The model under review builds one solid part; all positions refer to its coordinate system, in mm. A direction names the side the tool comes from. Round coordinates to 2 decimals unless told otherwise and drop trailing zeros. Order: outer loops, then holes, each group sorted by start corner. A loop starts at its lowest first (then second) coordinate and runs counter-clockwise, first axis right, second up. Notation, with made-up numbers: M 43.5,-32.5 L 50.5,-32.5 A12 ccw 50.5,-15.5 Z; hole C 63.5,87 d11. An arc over 180 degrees is marked long. Use a Markdown table: item, result. Add a question column.
1. The part is to be moulded in two halves that separate along Y. For faces 1 (the cylindrical face through (-2.57, 13.4, 19.79)), 2 (the flat face through (0, 20, 17)), 3 (the cylindrical face through (-7.43, 17.04, 8.44)), 4 (the cylindrical face through (7.91, 8.82, 2.46)), say which applies: +Y half, -Y half, draft (parallel to the pull), parting line (faces both ways), or undercut.
2. To check wall thickness, follow probe 1 along X at (y, z) = (7.5, 11); probe 2 along Y at (x, z) = (-10, 9.5); probe 3 along Z at (x, y) = (10.5, -12). State the ranges of each line that lie inside material, in increasing order.
3. Consider section C-C on z = 30. State the section outline as (x, y) points, then the cut area to 3 significant figures.
4. For faces 5 (the cylindrical face through (-2.57, -3.24, 5.6)), 6 (the cylindrical face through (7.986, 17.042, 31.586)), list the 3-axis set-ups (+Z, -Z, +X, -X, +Y, -Y) from which the entire face can be reached by the end or side of a thin tool; tool diameter is ignored.
5. Consider section A-A on y = 16. State the section outline as (x, z) points, then the cut area to 3 significant figures.
6. Consider section B-B on z = 23. State the section outline as (x, y) points, then the cut area to 3 significant figures.
7. Consider section D-D on x = 0.5. State the section outline as (y, z) points.
8. Insertion check: P1, Ø1.3, axis at x = 7.78, y = 7.78, coming from the -Z side; P2, Ø8, axis at x = -6.5, z = 18.5, coming from the -Y side; P3, Ø4, axis at x = -13, z = 22.5, coming from the -Y side; P4, Ø4, axis at x = 7, z = 15, coming from the -Y side. Each pin has a flat end and moves straight along its axis. Give the tip position at first contact, or say it passes through.
from build123d import *

# Parameters (mm, degrees)
SKETCH3_W                = 35
SKETCH3_H                = 40
BOSS_EXTRUDE1_DEPTH      = 5
SKETCH5_W                = 35
SKETCH5_H                = 30
BOSS_EXTRUDE2_DEPTH      = 6
BOSS_EXTRUDE3_DEPTH      = 4
BOSS_EXTRUDE4_DEPTH      = 2
BOSS_EXTRUDE4_DEPTH_BACK = 2
SKETCH9_R                = 1.05
CUT_EXTRUDE1_DEPTH       = 5
SKETCH10_R               = 1.6
CUT_EXTRUDE2_DEPTH       = 56.957573214
FILLET1_R                = 3
FILLET2_R                = 2


with BuildPart() as part:
    # Sketch3 → Boss-Extrude1 (new body)
    with BuildSketch(Plane.XY):
        Rectangle(SKETCH3_W, SKETCH3_H)
    extrude(amount=BOSS_EXTRUDE1_DEPTH)

    # Sketch5 → Boss-Extrude2 (add)
    with BuildSketch(Plane(origin=(0, 20, 0), x_dir=(1, 0, 0), z_dir=(0, 1, 0))):
        with Locations((0, -20)):
            Rectangle(SKETCH5_W, SKETCH5_H)
    extrude(amount=-BOSS_EXTRUDE2_DEPTH)

    # Sketch7 → Boss-Extrude3 (add)
    with BuildSketch(Plane(origin=(17.5, 0, 0), x_dir=(0, 0, -1), z_dir=(1, 0, 0))):
        Polygon((-35, 14), (-5, -20), (-5, 14), align=None)
    boss_extrude3 = extrude(amount=-BOSS_EXTRUDE3_DEPTH)

    # Mirror1: Boss-Extrude3 across plane
    add(boss_extrude3.mirror(Plane(origin=(0, 0, 0), x_dir=(0, 0, 1), z_dir=(1, 0, 0))))

    # Sketch8 → Boss-Extrude4 (add, two sides: drawn at the far end of the back side and taken through both)
    with BuildSketch(Plane(origin=(0, 0, 0), x_dir=(0, 0, -1), z_dir=(1, 0, 0)).offset(-BOSS_EXTRUDE4_DEPTH_BACK)):
        Polygon((-35, 14), (-5, -20), (-5, 14), align=None)
    extrude(amount=BOSS_EXTRUDE4_DEPTH + BOSS_EXTRUDE4_DEPTH_BACK)

    # Sketch9 → Cut-Extrude1 (cut)
    with BuildSketch(Plane(origin=(0, 0, 0), x_dir=(-1, 0, 0), z_dir=(0, 0, -1))):
        with Locations((-7.778174593, 7.778174593)):
            Circle(SKETCH9_R)
        with Locations((7.778174593, 7.778174593)):
            Circle(SKETCH9_R)
        with Locations((7.778174593, -7.778174593)):
            Circle(SKETCH9_R)
        with Locations((-7.778174593, -7.778174593)):
            Circle(SKETCH9_R)
    extrude(amount=-CUT_EXTRUDE1_DEPTH, mode=Mode.SUBTRACT)

    # Sketch10 → Cut-Extrude2 (cut, through all)
    with BuildSketch(Plane(origin=(0, 20, 0), x_dir=(1, 0, 0), z_dir=(0, 1, 0))):
        with Locations(Location((-7.778174593, -10, 0), (0, 0, 180))):
            Circle(SKETCH10_R)
        with Locations(Location((-7.778174593, -30, 0), (0, 0, 180))):
            Circle(SKETCH10_R)
        with Locations(Location((7.778174593, -30, 0), (0, 0, 180))):
            Circle(SKETCH10_R)
        with Locations(Location((7.778174593, -10, 0), (0, 0, 180))):
            Circle(SKETCH10_R)
    extrude(amount=-CUT_EXTRUDE2_DEPTH, mode=Mode.SUBTRACT)

    # Fillet1
    fillet1_edges = [part.edges().sort_by_distance(p)[0] for p in [
        (0, -20, 0),
        (-17.5, 0, 0),
        (17.5, 0, 0),
    ]]
    fillet(fillet1_edges, radius=FILLET1_R)

    # Fillet2
    # the kernel refuses this fillet: 2 mm, written as the material it adds along each edge
    with BuildSketch(Plane(origin=(13.5, 14, 0), x_dir=(0, -1, 0), z_dir=(0, 0, 1))) as fillet2_piece_1_section:
        with BuildLine():
            CenterArc((FILLET2_R, -FILLET2_R), FILLET2_R, 90, 90)
            Line((0, -FILLET2_R), (0, 0))
            Line((0, 0), (FILLET2_R, 0))
        make_face()
    fillet2_piece_1 = extrude(amount=35, mode=Mode.PRIVATE)
    fillet2_piece_1 = split(fillet2_piece_1, bisect_by=Plane(origin=(13.047209771, -2.378125245, 20.548713019), z_dir=(0, 0.6616216370868465, -0.7498378553650924)), keep=Keep.TOP, mode=Mode.PRIVATE)
    add(fillet2_piece_1)
    with BuildSketch(Plane(origin=(13.5, -20, 5), x_dir=(-1, 0, 0), z_dir=(0, 1, 0))) as fillet2_piece_2_section:
        with BuildLine():
            CenterArc((FILLET2_R, FILLET2_R), FILLET2_R, 180, 90)
            Line((0, FILLET2_R), (0, 0))
            Line((0, 0), (FILLET2_R, 0))
        make_face()
    fillet2_piece_2 = extrude(amount=39, mode=Mode.PRIVATE)
    fillet2_piece_2 = split(fillet2_piece_2, bisect_by=Plane(origin=(13.043521125, -10.077324079, 13.755302283), z_dir=(0, 0.6616216370868465, -0.7498378553650924)), keep=Keep.TOP, mode=Mode.PRIVATE)
    add(fillet2_piece_2)
    with BuildSketch(Plane(origin=(-13.5, 14, 0), x_dir=(0, -1, 0), z_dir=(0, 0, 1))) as fillet2_piece_3_section:
        with BuildLine():
            CenterArc((FILLET2_R, FILLET2_R), FILLET2_R, 180, 90)
            Line((0, FILLET2_R), (0, 0))
            Line((0, 0), (FILLET2_R, 0))
        make_face()
    fillet2_piece_3 = extrude(amount=35, mode=Mode.PRIVATE)
    fillet2_piece_3 = split(fillet2_piece_3, bisect_by=Plane(origin=(-13.047209771, -2.378125245, 20.548713019), z_dir=(0, 0.6616216370868465, -0.7498378553650924)), keep=Keep.TOP, mode=Mode.PRIVATE)
    add(fillet2_piece_3)
    with BuildSketch(Plane(origin=(-13.5, -20, 5), x_dir=(1, 0, 0), z_dir=(0, 1, 0))) as fillet2_piece_4_section:
        with BuildLine():
            CenterArc((FILLET2_R, -FILLET2_R), FILLET2_R, 90, 90)
            Line((0, -FILLET2_R), (0, 0))
            Line((0, 0), (FILLET2_R, 0))
        make_face()
    fillet2_piece_4 = extrude(amount=39, mode=Mode.PRIVATE)
    fillet2_piece_4 = split(fillet2_piece_4, bisect_by=Plane(origin=(-13.043521125, -10.077324079, 13.755302283), z_dir=(0, 0.6616216370868465, -0.7498378553650924)), keep=Keep.TOP, mode=Mode.PRIVATE)
    add(fillet2_piece_4)
    with BuildSketch(Plane(origin=(-2, 14, 0), x_dir=(-1, 0, 0), z_dir=(0, 0, 1))) as fillet2_piece_5_section:
        with BuildLine():
            CenterArc((FILLET2_R, FILLET2_R), FILLET2_R, 180, 90)
            Line((0, FILLET2_R), (0, 0))
            Line((0, 0), (FILLET2_R, 0))
        make_face()
    fillet2_piece_5 = extrude(amount=35, mode=Mode.PRIVATE)
    fillet2_piece_5 = split(fillet2_piece_5, bisect_by=Plane(origin=(-2.452790229, -2.378125245, 20.548713019), z_dir=(0, 0.6616216370868465, -0.7498378553650924)), keep=Keep.TOP, mode=Mode.PRIVATE)
    add(fillet2_piece_5)
    with BuildSketch(Plane(origin=(-2, -20, 5), x_dir=(-1, 0, 0), z_dir=(0, 1, 0))) as fillet2_piece_6_section:
        with BuildLine():
            CenterArc((FILLET2_R, FILLET2_R), FILLET2_R, 180, 90)
            Line((0, FILLET2_R), (0, 0))
            Line((0, 0), (FILLET2_R, 0))
        make_face()
    fillet2_piece_6 = extrude(amount=39, mode=Mode.PRIVATE)
    fillet2_piece_6 = split(fillet2_piece_6, bisect_by=Plane(origin=(-2.456478875, -10.077324079, 13.755302283), z_dir=(0, 0.6616216370868465, -0.7498378553650924)), keep=Keep.TOP, mode=Mode.PRIVATE)
    add(fillet2_piece_6)
    with BuildSketch(Plane(origin=(2, 14, 0), x_dir=(0, -1, 0), z_dir=(0, 0, 1))) as fillet2_piece_7_section:
        with BuildLine():
            CenterArc((FILLET2_R, FILLET2_R), FILLET2_R, 180, 90)
            Line((0, FILLET2_R), (0, 0))
            Line((0, 0), (FILLET2_R, 0))
        make_face()
    fillet2_piece_7 = extrude(amount=35, mode=Mode.PRIVATE)
    fillet2_piece_7 = split(fillet2_piece_7, bisect_by=Plane(origin=(2.452790229, -2.378125245, 20.548713019), z_dir=(0, 0.6616216370868465, -0.7498378553650924)), keep=Keep.TOP, mode=Mode.PRIVATE)
    add(fillet2_piece_7)
    with BuildSketch(Plane(origin=(2, -20, 5), x_dir=(1, 0, 0), z_dir=(0, 1, 0))) as fillet2_piece_8_section:
        with BuildLine():
            CenterArc((FILLET2_R, -FILLET2_R), FILLET2_R, 90, 90)
            Line((0, -FILLET2_R), (0, 0))
            Line((0, 0), (FILLET2_R, 0))
        make_face()
    fillet2_piece_8 = extrude(amount=39, mode=Mode.PRIVATE)
    fillet2_piece_8 = split(fillet2_piece_8, bisect_by=Plane(origin=(2.456478875, -10.077324079, 13.755302283), z_dir=(0, 0.6616216370868465, -0.7498378553650924)), keep=Keep.TOP, mode=Mode.PRIVATE)
    add(fillet2_piece_8)


solid = part.part
Answer block:
| question | item | result |
|---|---|---|
| 1 | face 1 | -Y half |
| 1 | face 2 | +Y half |
| 1 | face 3 | draft |
| 1 | face 4 | undercut |
| 2 | probe 1 | -17.5 to -13.5, -2 to 2, 13.5 to 17.5 |
| 2 | probe 2 | 14 to 20 |
| 2 | probe 3 | 0 to 5 |
| 3 | outline | M -17.5,8.33 L -13.5,8.33 L -13.5,12 A2 cw -11.5,14 L -9.38,14 L -9.38,20 L -17.5,20 Z; M -6.18,14 L -4,14 A2 cw -2,12 L -2,8.33 L 2,8.33 L 2,12 A2 cw 4,14 L 6.18,14 L 6.18,20 L -6.18,20 Z; M 9.38,14 L 11.5,14 A2 cw 13.5,12 L 13.5,8.33 L 17.5,8.33 L 17.5,20 L 9.38,20 Z |
| 3 | area | 243 mm^2 |
| 4 | face 5 | +Z, -Y |
| 4 | face 6 | +Y, -Y |
| 5 | outline | M -17.5,3 A3 ccw -14.5,0 L 14.5,0 A3 ccw 17.5,3 L 17.5,35 L -17.5,35 Z; hole C -7.78,10 d3.2; hole C -7.78,30 d3.2; hole C 7.78,10 d3.2; hole C 7.78,30 d3.2 |
| 5 | area | 1,190 mm^2 |
| 6 | outline | M -17.5,0.4 L -13.5,0.4 L -13.5,12 A2 cw -11.5,14 L -4,14 A2 cw -2,12 L -2,0.4 L 2,0.4 L 2,12 A2 cw 4,14 L 11.5,14 A2 cw 13.5,12 L 13.5,0.4 L 17.5,0.4 L 17.5,20 L -17.5,20 Z |
| 6 | area | 377 mm^2 |
| 7 | outline | M -20,3 A3 ccw -17,0 L 20,0 L 20,35 L 14,35 L -20,5 Z |
| 8 | P1 | through |
| 8 | P2 | y = 13.32 |
| 8 | P3 | y = -2.36 |
| 8 | P4 | y = 14 |
